The drawing under review shows one solid part. Ordinate dimensions are in mm from its lowest x, y, z. A direction names the side the tool comes from. Give positions to 0.01 mm unless a question says otherwise; leave off trailing zeros. Write each loop counter-clockwise with the first axis right and the second up, starting at its lowest first coordinate (ties: lowest second). Pieces come first, ordered by that corner, then holes. Notation, with made-up numbers: (72, 85) -> (129, 85) arc R13 ccw to (129, 90) -> close; hole circle Ø11 at (47.5, 28.25). An arc over 180 degrees is marked (long way). Use CSV: the item, a comma, the result in double quotes.
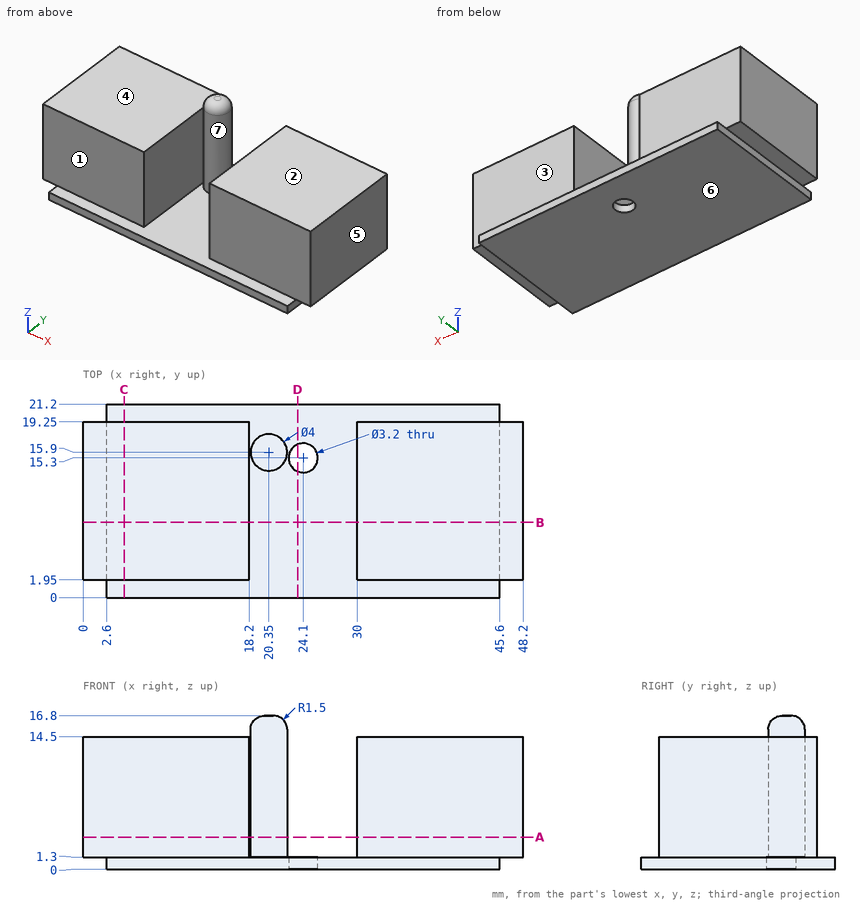
(1) Mouldability with a two-part tool opening along X and no side actions: class the marked faces 5, 6 and 7 as +X half, -X half, draft (parallel to the pull), parting line (faces both ways), or undercut.
Established:
face 5,"+X half"
face 6,"draft"
face 7,"undercut"
(2) Take a section at B-B (y = 8.25). Write out the cut boundary in (x, z).
Established:
outline,"(0, 1.3) -> (2.6, 1.3) -> (2.6, 0) -> (45.6, 0) -> (45.6, 1.3) -> (48.2, 1.3) -> (48.2, 14.5) -> (30, 14.5) -> (30, 1.3) -> (18.2, 1.3) -> (18.2, 14.5) -> (0, 14.5) -> close"
(3) Take a section at A-A (z = 3.5). Write out the cut boundary in (x, y), then the cut area to 3 significant figures.
Established:
outline,"(0, 1.95) -> (18.2, 1.95) -> (18.2, 19.25) -> (0, 19.25) -> close; circle Ø4 at (20.35, 15.9); (30, 1.95) -> (48.2, 1.95) -> (48.2, 19.25) -> (30, 19.25) -> close"
area,"642 mm2"
(4) For line 1 along X through (y, z) = (4.5, 11.25); line 2 along Y through (x, z) = (24.1, 1); line 3 along Y through (x, z) = (41, 6.25), list the stretches that pass through material, from the lowest coordinate up. Write a range as [from, to].
Established:
line 1,"x = [0, 18.2], [30, 48.2]"
line 2,"y = [0, 13.7], [16.9, 21.2]"
line 3,"y = [1.95, 19.25]"
(5) Clearance check with flat-ended pins moving along their axes: pin 1 (1 mm diameter, centred on x = 12.5, z = 2, fed in from +Y); pin 2 (5 mm diameter, centred on x = 37, y = 14.5, fed in from +Z); pin 3 (4 mm diameter, centred on x = 37.5, z = 8, fed in from -Y). State where each tip first meets the part, or that it passes through.
Established:
pin 1,"stops at y = 19.25"
pin 2,"stops at z = 14.5"
pin 3,"stops at y = 1.95"
(6) Tool access review of the marked faces 1, 2, 3 and 4: name each direction out of +Z, -Z, +X, -X, +Y, -Y from which nothing blocks a thin tool from reaching the whole face with its end or side.
Established:
face 1,"+Z, +X, -X, -Y"
face 2,"+Z, +X, +Y, -Y"
face 3,"+Z, +X, -X, +Y"
face 4,"+Z, -X, +Y, -Y"
(7) Take a section at D-D (x = 23.5). Write out the cut boundary in (y, z), then the cut area to 3 significant figures.
Established:
outline,"(0, 0) -> (13.82, 0) -> (13.82, 1.3) -> (0, 1.3) -> close; (16.78, 0) -> (21.2, 0) -> (21.2, 1.3) -> (16.78, 1.3) -> close"
area,"23.7 mm2"
(8) Take a section at C-C (x = 4.5). Write out the cut boundary in (y, z).
Established:
outline,"(0, 0) -> (21.2, 0) -> (21.2, 1.3) -> (19.25, 1.3) -> (19.25, 14.5) -> (1.95, 14.5) -> (1.95, 1.3) -> (0, 1.3) -> close"
